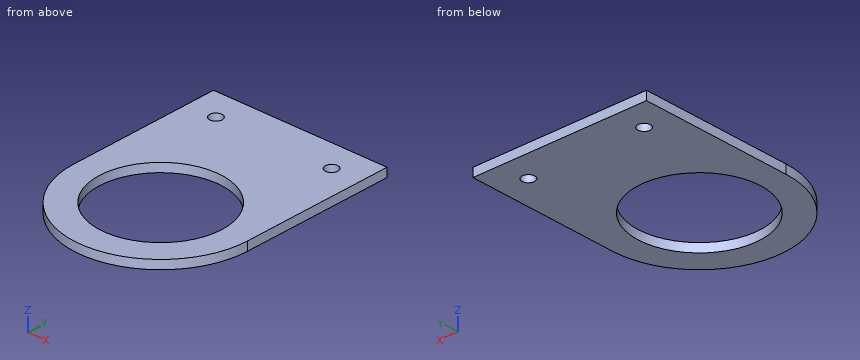
from build123d import *

# Parameters (mm, degrees)
SKETCH_1_R      = 21.15
SKETCH_1_R_2    = 2.15
EXTRUDE_1_DEPTH = 3


with BuildPart() as part:
    # 草图1 → 凸台-拉伸1 (new body)
    with BuildSketch(Plane.XY):
        with BuildLine():
            Line((-30, 0), (-30, 52.68))
            Line((-30, 52.68), (30, 52.68))
            Line((30, 52.68), (30, 0))
            ThreePointArc((30, 0), (0, -30), (-30, 0))
        make_face()
        Circle(SKETCH_1_R, mode=Mode.SUBTRACT)
        with Locations((-20, 42.68)):
            Circle(SKETCH_1_R_2, mode=Mode.SUBTRACT)
        with Locations((20, 42.68)):
            Circle(SKETCH_1_R_2, mode=Mode.SUBTRACT)
    extrude(amount=EXTRUDE_1_DEPTH)


solid = part.part
Model file for the job. Use its own axes, mm. Coordinates: 2 decimals unless noted, no trailing zeros. Write each loop counter-clockwise with the first axis right and the second up, starting at its lowest first coordinate (ties: lowest second). Pieces come first, ordered by that corner, then holes. Notation, with made-up numbers: (1.5, 48) - (49.5, 48) arc R9 ccw to (49.5, 65) - close; hole circle Ø8 at (-4.75, -27.75). An arc over 180 degrees is marked (long way). Write each question's results on one line, items separated by ' | '. Start each with the question number.
1) Cut at A-A (x = 0). Write the cut outline in (y, z), then the cut area to 3 significant figures.
2) Flat gauge pin, fed straight in: P1, Ø3.5, axis at x = -20, y = 42.68, coming from the +Z side. Where does the tip first touch, or does it go through?
3) Cut at B-B (y = 42.68). Write the cut outline in (x, z).
4) Probe line 1 along Y through (x, z) = (-18.5, 1.55); line 2 along X through (y, z) = (-1, 1.95); line 3 along X through (y, z) = (16.5, 0.7). List the from-to ranges inside material, lowest first. Write a range as from..to.
5) Cut at C-C (z = 0.65). Write the cut outline in (x, y), then the cut area to 3 significant figures.
6) Cut at D-D (x = -20). Write the cut outline in (y, z).
Returned:
1) outline: (-30, 0) - (-21.15, 0) - (-21.15, 3) - (-30, 3) - close; (21.15, 0) - (52.68, 0) - (52.68, 3) - (21.15, 3) - close | area: 121 mm^2
2) P1: through
3) outline: (-30, 0) - (-22.15, 0) - (-22.15, 3) - (-30, 3) - close; (-17.85, 0) - (17.85, 0) - (17.85, 3) - (-17.85, 3) - close; (22.15, 0) - (30, 0) - (30, 3) - (22.15, 3) - close
4) line 1: -23.62..-10.25, 10.25..41.14, 44.22..52.68 | line 2: -29.98..-21.13, 21.13..29.98 | line 3: -30..-13.23, 13.23..30
5) outline: (-30, 0) arc R30 ccw to (30, 0) - (30, 52.68) - (-30, 52.68) - close; hole circle Ø4.3 at (-20, 42.68); hole circle Ø42.3 at (0, 0); hole circle Ø4.3 at (20, 42.68) | area: 3,140 mm^2
6) outline: (-22.36, 0) - (-6.88, 0) - (-6.88, 3) - (-22.36, 3) - close; (6.88, 0) - (40.53, 0) - (40.53, 3) - (6.88, 3) - close; (44.83, 0) - (52.68, 0) - (52.68, 3) - (44.83, 3) - close
